For this review, take the finished solid that the model builds, in its own axes (mm). A direction names the side the tool comes from. Round coordinates to 2 decimals unless told otherwise and drop trailing zeros. Loops run counter-clockwise (first coordinate to the right, second up) from the corner with the lowest first, then second, coordinate; pieces in that order, holes last.
```python
from build123d import *

# Parameters (mm, degrees)
ESQUISSE1_R             = 2.5
ESQUISSE1_R_2           = 0.6
BOSS_EXTRU_1_DEPTH      = 1
ENL_V_MAT_EXTRU_1_DEPTH = 15.899664426
BOSS_EXTRU_2_DEPTH      = 0.5
BOSS_EXTRU_3_DEPTH      = 0.5


with BuildPart() as part:
    # Esquisse1 → Boss.-Extru.1 (new body)
    with BuildSketch(Plane.XY):
        with BuildLine():
            Line((-8.351646544, 5.5), (8.351646544, 5.5))
            ThreePointArc((8.351646544, 5.5), (9.995328218, -0.30563675), (8, -6))
            Line((8, -6), (8, -11))
            Line((8, -11), (-8, -11))
            Line((-8, -11), (-8, -6))
            ThreePointArc((-8, -6), (-9.995328218, -0.30563675), (-8.351646544, 5.5))
        make_face()
        Circle(ESQUISSE1_R, mode=Mode.SUBTRACT)
        with Locations((-6.4, -9.6)):
            Circle(ESQUISSE1_R_2, mode=Mode.SUBTRACT)
        with Locations((-3.84, -9.6)):
            Circle(ESQUISSE1_R_2, mode=Mode.SUBTRACT)
        with Locations((-1.28, -9.6)):
            Circle(ESQUISSE1_R_2, mode=Mode.SUBTRACT)
        with Locations((1.28, -9.6)):
            Circle(ESQUISSE1_R_2, mode=Mode.SUBTRACT)
        with Locations((3.84, -9.6)):
            Circle(ESQUISSE1_R_2, mode=Mode.SUBTRACT)
        with Locations((6.4, -9.6)):
            Circle(ESQUISSE1_R_2, mode=Mode.SUBTRACT)
        with BuildLine():
            Line((-6.3, 0.8), (-6.3, -1.444183839))
            ThreePointArc((-6.3, -1.444183839), (-6.419746949, -1.690835185), (-6.641967863, -1.851440553))
            Line((-6.641967863, -1.851440553), (-8.292953638, -2.509553847))
            ThreePointArc((-8.292953638, -2.509553847), (-9.009553847, -2.207046362), (-8.707046362, -1.490446153))
            Line((-8.707046362, -1.490446153), (-7.4, -0.969433434))
            Line((-7.4, -0.969433434), (-7.4, 0.8))
            ThreePointArc((-7.4, 0.8), (-6.85, 1.370822155), (-6.3, 0.8))
        make_face(mode=Mode.SUBTRACT)
        with BuildLine():
            Line((7.4, 1.315402872), (7.4, -1))
            ThreePointArc((7.4, -1), (6.85, -1.55), (6.3, -1))
            Line((6.3, -1), (6.3, 1.315402872))
            ThreePointArc((6.3, 1.315402872), (6.85, 1.865402872), (7.4, 1.315402872))
        make_face(mode=Mode.SUBTRACT)
    extrude(amount=BOSS_EXTRU_1_DEPTH)

    # Esquisse2 → Enlèv. mat.-Extru.1 (cut, through all)
    with BuildSketch(Plane.XY.offset(1)):
        with BuildLine():
            Line((6.668307266, 1.834524968), (8.317330789, 2.411683201))
            ThreePointArc((8.317330789, 2.411683201), (9.018145619, 2.074253838), (8.680716257, 1.373439009))
            Line((8.680716257, 1.373439009), (7.031692734, 0.796280776))
            ThreePointArc((7.031692734, 0.796280776), (6.330877904, 1.133710138), (6.668307266, 1.834524968))
        make_face()
    extrude(amount=-ENL_V_MAT_EXTRU_1_DEPTH, mode=Mode.SUBTRACT)

    # Esquisse3 → Boss.-Extru.2 (add)
    with BuildSketch(Plane.XY.offset(1)):
        Polygon((-4.950824849, 3.498836933), (-2.906168647, 1.454180731), (-1.81491955, 2.545429827), (-3.859575753, 4.59008603), align=None)
    extrude(amount=BOSS_EXTRU_2_DEPTH)

    # Esquisse4 → Boss.-Extru.3 (add)
    with BuildSketch(Plane.XY.offset(1)):
        Polygon((1.711538057, 2.510969329), (3.767681092, 4.567112364), (4.853186772, 3.481606684), (2.797043737, 1.425463649), align=None)
    extrude(amount=BOSS_EXTRU_3_DEPTH)


solid = part.part
```
(1) Add section A-A (x = 0). Give the boundary of the cut face in (y, z).
(2) The part is to be moulded in two halves that separate along X. For faces 1 (the flat face through (0.1, -11, 0.5)), 2 (the cylindrical face through (10, -0.2, 0.5)), 3 (the flat face through (-8.063, -1.234, 0.493)), say which applies: pulls with the +X half, pulls with the -X half, needs draft (parallel to the pull), parting line crosses it, or undercut.
(3) Add section C-C (y = -6.75). Give the boundary of the cut face in (x, z), plus the area to 3 significant figures.
(4) Insertion check: pin 1 Ø0.5 at (y, z) = (0.5, 0.5) entering from -X; pin 2 Ø1 at (x, y) = (-1.28, -9.6) entering from -Z; pin 3 Ø0.5 at (y, z) = (-7.5, 0.5) entering from +X; pin 4 Ø8 at (x, y) = (0, 0) entering from -Z. Each pin has a flat end and moves straight along its axis. Give the tip position at first contact, or say it passes through.
(5) For faces 4 (the flat face through (2.26, 1.96, 1.25)), 5 (the flat face through (2.7, 3.5, 1.2)), 6 (the cylindrical face through (-6.86, 1.37, 0.49)), list the 3-axis set-ups (+Z, -Z, +X, -X, +Y, -Y) from which the entire face can be reached by the end or side of a thin tool; tool diameter is ignored.
(6) For L1, parallel to Y at x = 3.84, z = 0.4; L2, parallel to X at y = -0.5, z = 0.5; L3, parallel to Z at x = -3, y = -1.25, list the stretches that pass through material, from the lowest coordinate up.
(7) Add section B-B (z = 0.7). Give the number of separate pieces and of enclosed holes in the cut face, plus the area to 3 significant figures.
Outcome:
1. outline: (-11, 0) - (-2.5, 0) - (-2.5, 1) - (-11, 1) - close; (2.5, 0) - (5.5, 0) - (5.5, 1) - (2.5, 1) - close
2. face 1: needs draft
2. face 2: pulls with the +X half
2. face 3: undercut
3. outline: (-8, 0) - (8, 0) - (8, 1) - (-8, 1) - close
3. area: 16.0 mm2
4. pin 1: stops at x = -10
4. pin 2: passes through
4. pin 3: stops at x = 8
4. pin 4: stops at z = 0
5. face 4: +Z, -Y
5. face 5: +Z, +Y
5. face 6: +Z, -Z
6. L1: y = -11 to -10.2, -9 to 5.5
6. L2: x = -9.99 to -7.4, -6.3 to -2.45, 2.45 to 6.3, 7.4 to 9.99
6. L3: z = 0 to 1
7. separate pieces: 1
7. enclosed holes: 9
7. area: 259 mm2
